```python
from build123d import *

# Parameters (mm, degrees)
SKETCH1_R           = 20
SKETCH1_R_2         = 16
BOSS_EXTRUDE1_DEPTH = 350
SKETCH2_W           = 46.702536181
SKETCH2_H           = 100
CUT_EXTRUDE1_DEPTH  = 100
SKETCH3_W           = 194.995303171
SKETCH3_H           = 10.817431772
BOSS_EXTRUDE2_DEPTH = 105.29
SKETCH4_W           = 194.995303171
SKETCH4_H           = 100
BOSS_EXTRUDE3_DEPTH = 20
CHAMFER1_SIZE       = 10
FILLET1_R           = 5
SKETCH5_W           = 100
SKETCH5_H           = 20
BOSS_EXTRUDE4_DEPTH = 6


with BuildPart() as part:
    # Sketch1 → Boss-Extrude1 (new, symmetric)
    with BuildSketch(Plane.XY):
        Circle(SKETCH1_R)
        Circle(SKETCH1_R_2, mode=Mode.SUBTRACT)
    extrude(amount=BOSS_EXTRUDE1_DEPTH, both=True)

    # Sketch2 → Cut-Extrude1 (cut, symmetric)
    with BuildSketch(Plane(origin=(0, 0, 0), x_dir=(1, 0, 0), z_dir=(0, 1, 0))):
        with Locations((-23.351268091, -220)):
            Rectangle(SKETCH2_W, SKETCH2_H)
    extrude(amount=CUT_EXTRUDE1_DEPTH, both=True, mode=Mode.SUBTRACT)

    # Sketch3 → Boss-Extrude2 (add)
    with BuildSketch(Plane(origin=(0, 0, 0), x_dir=(0, 0, -1), z_dir=(1, 0, 0))):
        with Locations((-234.028576152, 0)):
            Rectangle(SKETCH3_W, SKETCH3_H)
    extrude(amount=BOSS_EXTRUDE2_DEPTH)

    # Sketch4 → Boss-Extrude3 (add)
    with BuildSketch(Plane(origin=(105.29, 0, 0), x_dir=(0, 0, -1), z_dir=(1, 0, 0))):
        with Locations((-234.028576152, 0)):
            Rectangle(SKETCH4_W, SKETCH4_H)
    extrude(amount=-BOSS_EXTRUDE3_DEPTH)

    # Chamfer1
    chamfer1_edges = [part.edges().sort_by_distance(p)[0] for p in [
        (85.29, -5.408715886, 234.028576151),
        (85.29, 5.408715886, 234.028576151),
    ]]
    chamfer(chamfer1_edges, length=CHAMFER1_SIZE)

    # Fillet1
    fillet1_edges = [part.edges().sort_by_distance(p)[0] for p in [
        (95.29, 50, 136.530924566),
        (95.29, -50, 331.526227737),
        (95.29, -50, 136.530924566),
        (95.29, 50, 331.526227737),
    ]]
    fillet(fillet1_edges, radius=FILLET1_R)

    # Sketch5 → Boss-Extrude4 (add)
    with BuildSketch(Plane.ZY):
        with Locations((220, 26)):
            Rectangle(SKETCH5_W, SKETCH5_H)
        with Locations((220, -26)):
            Rectangle(SKETCH5_W, SKETCH5_H)
    extrude(amount=-BOSS_EXTRUDE4_DEPTH)


solid = part.part
```
Work out the finished part from the listing and answer in its coordinate system (mm). A direction names the side the tool comes from. Coordinates: 2 decimals unless noted, no trailing zeros. Loops run counter-clockwise (first coordinate to the right, second up) from the corner with the lowest first, then second, coordinate; pieces in that order, holes last.
1) Section B-B (z = 160) is taken. Give the vertices of the cut face in (x, y), plus the area to 3 significant figures.
Results:
outline: (19.25, -5.41) - (75.29, -5.41) - (85.29, -15.41) - (85.29, -50) - (105.29, -50) - (105.29, 50) - (85.29, 50) - (85.29, 15.41) - (75.29, 5.41) - (19.25, 5.41) arc R20 ccw (long way) to start; hole (0, -5.41) - (0, 5.41) - (15.06, 5.41) arc R16 ccw (long way) to (15.06, -5.41) - close
area: 3,430 mm2
2) Flat-ended cylindrical pins translate along their axes: pin 1 (5 mm diameter, centred on y = -9.5, z = 80.5, fed in from -X) (3 decimals); pin 2 (3 mm diameter, centred on y = 1, z = 269.5, fed in from -X); pin 3 (16.5 mm diameter, centred on x = 4, z = 250.5, fed in from -Y). Find the tip coordinate at first contact, or state that the pin passes through.
Results:
pin 1: stops at x = -18.735
pin 2: stops at x = -20
pin 3: stops at y = -36
3) Section D-D (z = 66.5) is taken. Give the vertices of the cut face in (x, y).
Results:
outline: circle Ø40 at (0, 0); hole circle Ø32 at (0, 0)
4) Consider probe 1 along X at (y, z) = (0, 53.5); probe 2 along X at (y, z) = (1.5, 47.5). Determine where each line is inside the solid, lowest interval first.
Results:
probe 1: x = -20 to -16, 16 to 20
probe 2: x = -19.94 to -15.93, 15.93 to 19.94
5) For faces 4 (the flat face through (82, 0, 331.526)), 5 (the flat face through (-17, -1, 270)), 6 (the flat face through (6, 28, 219)), 7 (the flat face through (6, -27, 219)), determine the directions among +Z, -Z, +X, -X, +Y, -Y from which every point of the face is accessible in a straight line to the end or side of a thin tool.
Results:
face 4: +Z, +X, +Y, -Y
face 5: -X, +Y, -Y
face 6: +Z, -Z, +Y
face 7: +Z, -Z, -Y
6) Section A-A (y = -29.5) is taken. Give the vertices of the cut face in (x, z), plus the area to 3 significant figures.
Results:
outline: (0, 170) - (6, 170) - (6, 270) - (0, 270) - close; (85.29, 136.53) - (105.29, 136.53) - (105.29, 331.53) - (85.29, 331.53) - close
area: 4,500 mm2
7) Section C-C (x = 67) is taken. Give the vertices of the cut face in (y, z).
Results:
outline: (-5.41, 136.53) - (5.41, 136.53) - (5.41, 331.53) - (-5.41, 331.53) - close
8) For a pull along Z with two mould halves and no side action, classify faces 1 (the flat face through (-8.98, 13.43, -350)), 2 (the flat face through (-17, -1, 170)), 3 (the flat face through (-8.98, 13.43, 350)) as +Z half, -Z half, draft (parallel to the pull), parting line (faces both ways), or undercut.
Results:
face 1: -Z half
face 2: undercut
face 3: +Z half
